from build123d import *

# Parameters (mm, degrees)
SKETCH1_R           = 3
BOSS_EXTRUDE1_DEPTH = 1.5
SKETCH2_R           = 2.4
BOSS_EXTRUDE2_DEPTH = 1.25
SKETCH4_R           = 3
BOSS_EXTRUDE3_DEPTH = 6.2
CUT_EXTRUDE1_START  = -6.2
CUT_EXTRUDE1_DEPTH  = 6.2
SKETCH6_W           = 1.25
SKETCH6_H           = 6
CUT_EXTRUDE2_DEPTH  = 7.45


with BuildPart() as part:
    # Sketch1 → Boss-Extrude1 (new body)
    with BuildSketch(Plane(origin=(0, 0, 0), x_dir=(1, 0, 0), z_dir=(0, 1, 0))):
        with Locations(Location((0, 0, 0), (0, 0, 270))):
            Circle(SKETCH1_R)
    extrude(amount=BOSS_EXTRUDE1_DEPTH)

    # Sketch2 → Boss-Extrude2 (add)
    with BuildSketch(Plane(origin=(0, 1.5, 0), x_dir=(1, 0, 0), z_dir=(0, 1, 0))):
        with Locations(Location((0, 0, 0), (0, 0, 270))):
            Circle(SKETCH2_R)
    extrude(amount=BOSS_EXTRUDE2_DEPTH)

    # Sketch4 → Boss-Extrude3 (add)
    with BuildSketch(Plane(origin=(0, 2.75, 0), x_dir=(1, 0, 0), z_dir=(0, 1, 0))):
        with Locations(Location((0, 0, 0), (0, 0, 270))):
            Circle(SKETCH4_R)
    extrude(amount=BOSS_EXTRUDE3_DEPTH)

    # Sketch5 → Cut-Extrude1 (cut)
    with BuildSketch(Plane(origin=(0, 8.95, 0), x_dir=(1, 0, 0), z_dir=(0, 1, 0)).offset(CUT_EXTRUDE1_START)):
        with BuildLine():
            Line((-0.489527377, 2.461020315), (0, 3))
            ThreePointArc((0, 3), (-0.585270966, 2.942355841), (-1.148050297, 2.771638598))
            Line((-1.148050297, 2.771638598), (-0.489527377, 2.461020315))
        make_face()
        with BuildLine():
            Line((-1.394056026, 2.086352282), (-1.148050297, 2.771638598))
            ThreePointArc((-1.148050297, 2.771638598), (-1.666710699, 2.494408837), (-2.121320344, 2.121320344))
            Line((-2.121320344, 2.121320344), (-1.394056026, 2.086352282))
        make_face()
        with BuildLine():
            Line((-2.086352282, 1.394056026), (-2.121320344, 2.121320344))
            ThreePointArc((-2.121320344, 2.121320344), (-2.494408837, 1.666710699), (-2.771638598, 1.148050297))
            Line((-2.771638598, 1.148050297), (-2.086352282, 1.394056026))
        make_face()
        with BuildLine():
            Line((-2.461020315, 0.489527377), (-2.771638598, 1.148050297))
            ThreePointArc((-2.771638598, 1.148050297), (-2.942355841, 0.585270966), (-3, 0))
            Line((-3, 0), (-2.461020315, 0.489527377))
        make_face()
        with BuildLine():
            ThreePointArc((-3, 0), (-2.942355841, -0.585270966), (-2.771638598, -1.148050297))
            Line((-2.771638598, -1.148050297), (-2.461020315, -0.489527377))
            Line((-2.461020315, -0.489527377), (-3, 0))
        make_face()
        with BuildLine():
            ThreePointArc((-2.771638598, -1.148050297), (-2.494408837, -1.666710699), (-2.121320344, -2.121320344))
            Line((-2.121320344, -2.121320344), (-2.086352282, -1.394056026))
            Line((-2.086352282, -1.394056026), (-2.771638598, -1.148050297))
        make_face()
        with BuildLine():
            ThreePointArc((-2.121320344, -2.121320344), (-1.666710699, -2.494408837), (-1.148050297, -2.771638598))
            Line((-1.148050297, -2.771638598), (-1.394056026, -2.086352282))
            Line((-1.394056026, -2.086352282), (-2.121320344, -2.121320344))
        make_face()
        with BuildLine():
            ThreePointArc((-1.148050297, -2.771638598), (-0.585270966, -2.942355841), (0, -3))
            Line((0, -3), (-0.489527377, -2.461020315))
            Line((-0.489527377, -2.461020315), (-1.148050297, -2.771638598))
        make_face()
        with BuildLine():
            ThreePointArc((0, -3), (0.585270966, -2.942355841), (1.148050297, -2.771638598))
            Line((1.148050297, -2.771638598), (0.489527377, -2.461020315))
            Line((0.489527377, -2.461020315), (0, -3))
        make_face()
        with BuildLine():
            ThreePointArc((1.148050297, -2.771638598), (1.666710699, -2.494408837), (2.121320344, -2.121320344))
            Line((2.121320344, -2.121320344), (1.394056026, -2.086352282))
            Line((1.394056026, -2.086352282), (1.148050297, -2.771638598))
        make_face()
        with BuildLine():
            ThreePointArc((2.121320344, -2.121320344), (2.494408837, -1.666710699), (2.771638598, -1.148050297))
            Line((2.771638598, -1.148050297), (2.086352282, -1.394056026))
            Line((2.086352282, -1.394056026), (2.121320344, -2.121320344))
        make_face()
        with BuildLine():
            ThreePointArc((2.771638598, -1.148050297), (2.942355841, -0.585270966), (3, 0))
            Line((3, 0), (2.461020315, -0.489527377))
            Line((2.461020315, -0.489527377), (2.771638598, -1.148050297))
        make_face()
        with BuildLine():
            Line((2.461020315, 0.489527377), (3, 0))
            ThreePointArc((3, 0), (2.942355841, 0.585270966), (2.771638598, 1.148050297))
            Line((2.771638598, 1.148050297), (2.461020315, 0.489527377))
        make_face()
        with BuildLine():
            Line((2.086352282, 1.394056026), (2.771638598, 1.148050297))
            ThreePointArc((2.771638598, 1.148050297), (2.494408837, 1.666710699), (2.121320344, 2.121320344))
            Line((2.121320344, 2.121320344), (2.086352282, 1.394056026))
        make_face()
        with BuildLine():
            Line((1.394056026, 2.086352282), (2.121320344, 2.121320344))
            ThreePointArc((2.121320344, 2.121320344), (1.666710699, 2.494408837), (1.148050297, 2.771638598))
            Line((1.148050297, 2.771638598), (1.394056026, 2.086352282))
        make_face()
        with BuildLine():
            Line((0.489527377, 2.461020315), (1.148050297, 2.771638598))
            ThreePointArc((1.148050297, 2.771638598), (0.585270966, 2.942355841), (0, 3))
            Line((0, 3), (0.489527377, 2.461020315))
        make_face()
    extrude(amount=CUT_EXTRUDE1_DEPTH, mode=Mode.SUBTRACT)

    # Sketch6 → Cut-Extrude2 (cut)
    with BuildSketch(Plane(origin=(0, 8.95, 0), x_dir=(1, 0, 0), z_dir=(0, 1, 0))):
        Rectangle(SKETCH6_W, SKETCH6_H)
    extrude(amount=-CUT_EXTRUDE2_DEPTH, mode=Mode.SUBTRACT)


solid = part.part
Build history of the part. All positions in model axes, mm. A direction names the side the tool comes from. Give positions to 0.01 mm unless a question says otherwise; leave off trailing zeros. Order: outer loops, then holes, each group sorted by start corner. A loop starts at its lowest first (then second) coordinate and runs counter-clockwise, first axis right, second up. Notation, with made-up numbers: M 21.5,10.5 L 36.5,10.5 A14 cw 36.5,14.5 Z; hole C -25,33 d4. An arc over 180 degrees is marked long. Put each result on its own line as item: value.
Item 1: Pull direction X, two halves, no side cores. Call faces 1 (the face through (-2, 8.95, 0)), 2 (the face through (0, 1.5, 0)), 3 (the face through (0.9, 0.74, 2.86)): +X half, -X half, draft (parallel to the pull), parting line (faces both ways), or undercut.
Results are:
face 1: draft
face 2: undercut
face 3: parting line
Item 2: Drop a flat-ended pin along its axis: pin 1 Ø1 at (y, z) = (3, -1) entering from +X. Give the stop position or say it passes through.
Results are:
pin 1: x = 2.77
Item 3: Cut at C-C on y = 2.5. Write the cut outline in (x, z) (3 decimals), then the cut area to 3 significant figures.
Results are:
outline: M -0.625,-2.317 L -0.625,2.317 A2.4 ccw Z; M 0.625,-2.317 A2.4 ccw 0.625,2.317 Z
area: 12.2 mm2
Item 4: Cut at B-B on x = -0.9. Write the cut outline in (y, z), then the cut area to 3 significant figures.
Results are:
outline: M 0,-2.86 L 1.5,-2.86 L 1.5,-2.22 L 2.75,-2.22 L 2.75,-2.65 L 8.95,-2.65 L 8.95,2.65 L 2.75,2.65 L 2.75,2.22 L 1.5,2.22 L 1.5,2.86 L 0,2.86 Z
area: 47.1 mm2
Item 5: Wall check: probe 1 along Y at (x, z) = (-1, 2.3); probe 2 along X at (y, z) = (3.25, 1.5) (3 decimals); probe 3 along X at (y, z) = (4.25, 2.3) (3 decimals). Give the ranges that are in metal, low to high.
Results are:
probe 1: 0 to 1.5, 2.75 to 8.95
probe 2: -2.091 to -0.625, 0.625 to 2.091
probe 3: -1.317 to -0.625, 0.625 to 1.317
Item 6: Cut at D-D on x = -1.55. Write the cut outline in (y, z), then the cut area to 3 significant figures.
Results are:
outline: M 0,-2.57 L 1.5,-2.57 L 1.5,-1.83 L 2.75,-1.83 L 2.75,-2.09 L 8.95,-2.09 L 8.95,2.09 L 2.75,2.09 L 2.75,1.83 L 1.5,1.83 L 1.5,2.57 L 0,2.57 Z
area: 38.3 mm2
Item 7: Which spindle directions (+Z, -Z, +X, -X, +Y, -Y) get a long thin tool onto all of the face, cutting with end or side? Do faces 4 (the face through (0.625, 5, 0)), 5 (the face through (2, 8.95, 0)), 6 (the face through (-2.4, 2.1, 0)), 7 (the face through (2.4, 2.1, 0)). Say none if no direction does.
Results are:
face 4: +Z, -Z, +Y
face 5: +Z, -Z, +X, -X, +Y
face 6: -X
face 7: +X
